```python
from build123d import *

# Parameters (mm, degrees)
SKETCH1_W           = 153
SKETCH1_H           = 100
SKETCH1_R           = 3.25
BOSS_EXTRUDE1_DEPTH = 3.175
CUT_EXTRUDE1_DEPTH  = 92.4457797
CUT_EXTRUDE2_DEPTH  = 92.4457797
FILLET1_R           = 5
SKETCH4_R           = 1.25
CUT_EXTRUDE3_DEPTH  = 92.4457797
SKETCH5_R           = 1.25
CUT_EXTRUDE4_DEPTH  = 92.4457797
SKETCH6_W           = 85
SKETCH6_H           = 12.5
CUT_EXTRUDE5_DEPTH  = 92.4457797


with BuildPart() as part:
    # Sketch1 → Boss-Extrude1 (new body)
    with BuildSketch(Plane(origin=(0, 0, 0), x_dir=(1, 0, 0), z_dir=(0, 1, 0))):
        Rectangle(SKETCH1_W, SKETCH1_H)
        with Locations(Location((-70, 43.5, 0), (0, 0, 270))):
            Circle(SKETCH1_R, mode=Mode.SUBTRACT)
        with Locations(Location((70, 43.5, 0), (0, 0, 270))):
            Circle(SKETCH1_R, mode=Mode.SUBTRACT)
        with Locations(Location((70, -43.5, 0), (0, 0, 270))):
            Circle(SKETCH1_R, mode=Mode.SUBTRACT)
        with Locations(Location((-70, -43.5, 0), (0, 0, 270))):
            Circle(SKETCH1_R, mode=Mode.SUBTRACT)
    extrude(amount=BOSS_EXTRUDE1_DEPTH)

    # Sketch2 → Cut-Extrude1 (cut, through all)
    with BuildSketch(Plane(origin=(0, 3.175, 0), x_dir=(1, 0, 0), z_dir=(0, 1, 0))):
        Polygon((-76.5, 35), (-66.5, 35), (-45, 13.5), (-45, -13.5), (-66.5, -35), (-76.5, -35), align=None)
        Polygon((76.5, -35), (66.5, -35), (45, -13.5), (45, 13.5), (66.5, 35), (76.5, 35), align=None)
    extrude(amount=-CUT_EXTRUDE1_DEPTH, mode=Mode.SUBTRACT)

    # Sketch3 → Cut-Extrude2 (cut, through all)
    with BuildSketch(Plane(origin=(0, 3.175, 0), x_dir=(1, 0, 0), z_dir=(0, 1, 0))):
        with BuildLine():
            Line((-50, 45), (-50, 60))
            ThreePointArc((-50, 60), (-42.5, 67.5), (-35, 60))
            Line((-35, 60), (-35, 45))
            ThreePointArc((-35, 45), (-42.5, 37.5), (-50, 45))
        make_face()
        with BuildLine():
            Line((50, 45), (50, 60))
            ThreePointArc((50, 60), (42.5, 67.5), (35, 60))
            Line((35, 60), (35, 45))
            ThreePointArc((35, 45), (42.5, 37.5), (50, 45))
        make_face()
        with BuildLine():
            Line((-50, -45), (-50, -60))
            ThreePointArc((-50, -60), (-42.5, -67.5), (-35, -60))
            Line((-35, -60), (-35, -45))
            ThreePointArc((-35, -45), (-42.5, -37.5), (-50, -45))
        make_face()
        with BuildLine():
            Line((50, -45), (50, -60))
            ThreePointArc((50, -60), (42.5, -67.5), (35, -60))
            Line((35, -60), (35, -45))
            ThreePointArc((35, -45), (42.5, -37.5), (50, -45))
        make_face()
    extrude(amount=-CUT_EXTRUDE2_DEPTH, mode=Mode.SUBTRACT)

    # Fillet1
    fillet1_edges = [part.edges().sort_by_distance(p)[0] for p in [
        (-45, 1.5875, -13.5),
        (-45, 1.5875, 13.5),
        (-66.5, 1.5875, 35),
        (-50, 1.5875, 50),
        (-35, 1.5875, 50),
        (35, 1.5875, 50),
        (50, 1.5875, 50),
        (66.5, 1.5875, 35),
        (45, 1.5875, 13.5),
        (45, 1.5875, -13.5),
        (66.5, 1.5875, -35),
        (50, 1.5875, -50),
        (35, 1.5875, -50),
        (-35, 1.5875, -50),
        (-50, 1.5875, -50),
        (-66.5, 1.5875, -35),
    ]]
    fillet(fillet1_edges, radius=FILLET1_R - 0.0001)  # a hair under: the kernel refuses the full size

    # Sketch4 → Cut-Extrude3 (cut, through all)
    with BuildSketch(Plane(origin=(0, 3.175, 0), x_dir=(1, 0, 0), z_dir=(0, 1, 0))):
        with Locations(Location((-32.76, 10, 0), (0, 0, 270))):
            Circle(SKETCH4_R)
        with Locations(Location((-14.76, 22, 0), (0, 0, 270))):
            Circle(SKETCH4_R)
        with Locations(Location((-14.76, -22, 0), (0, 0, 270))):
            Circle(SKETCH4_R)
        with Locations(Location((-32.76, -22, 0), (0, 0, 270))):
            Circle(SKETCH4_R)
        with Locations(Location((32.76, -22, 0), (0, 0, 90))):
            Circle(SKETCH4_R)
        with Locations(Location((14.76, -22, 0), (0, 0, 90))):
            Circle(SKETCH4_R)
        with Locations(Location((14.76, 22, 0), (0, 0, 90))):
            Circle(SKETCH4_R)
        with Locations(Location((32.76, 10, 0), (0, 0, 90))):
            Circle(SKETCH4_R)
    extrude(amount=-CUT_EXTRUDE3_DEPTH, mode=Mode.SUBTRACT)

    # Sketch5 → Cut-Extrude4 (cut, through all)
    with BuildSketch(Plane(origin=(0, 3.175, 0), x_dir=(1, 0, 0), z_dir=(0, 1, 0))):
        with Locations(Location((-5, -10, 0), (0, 0, 270))):
            Circle(SKETCH5_R)
        with Locations(Location((5, -10, 0), (0, 0, 270))):
            Circle(SKETCH5_R)
    extrude(amount=-CUT_EXTRUDE4_DEPTH, mode=Mode.SUBTRACT)

    # Sketch6 → Cut-Extrude5 (cut, through all)
    with BuildSketch(Plane(origin=(0, 3.175, 0), x_dir=(1, 0, 0), z_dir=(0, 1, 0))):
        with Locations((0, 43.75)):
            Rectangle(SKETCH6_W, SKETCH6_H)
        with Locations((0, -43.75)):
            Rectangle(SKETCH6_W, SKETCH6_H)
    extrude(amount=-CUT_EXTRUDE5_DEPTH, mode=Mode.SUBTRACT)


solid = part.part
```
Input: part model. Units: mm. Frame: model coordinates. A direction names the side the tool comes from. Give positions to 0.01 mm unless a question says otherwise; leave off trailing zeros. Loops run counter-clockwise (first coordinate to the right, second up) from the corner with the lowest first, then second, coordinate; pieces in that order, holes last. Notation, with made-up numbers: (41.25, -15.5) -> (58.25, -15.5) arc R32 cw to (58.25, 17.5) -> close; hole circle Ø9 at (83, 60). An arc over 180 degrees is marked (long way). Use a Markdown table: item, result.
Q1. Access query for faces 1 (the flat face through (-1, 2, -37.5)), 2 (the cylindrical face through (-52, 2, 49)), 3 (the flat face through (-55.6, 1.6, 24.1)), 4 (the cylindrical face through (66.63, 1.57, 34.61)). Directions: +Z, -Z, +X, -X, +Y, -Y. A direction counts if a zero-diameter tool reaches every point of the face in a straight line with its end or side. Return the directions, or none.
Entries:
| item | result |
|---|---|
| face 1 | -Z, +Y, -Y |
| face 2 | +Z, +Y, -Y |
| face 3 | -X, +Y, -Y |
| face 4 | +X, +Y, -Y |
Q2. Section query B-B, the plane y = 2.25. State how many separate pieces and enclosed holes the cut face has, plus the area to 3 significant figures.
Entries:
| item | result |
|---|---|
| separate pieces | 1 |
| enclosed holes | 14 |
| area | 9,160 mm² |
Q3. Section query C-C, the plane x = 12. Return the cut outline in (y, z) (3 decimals).
Entries:
| item | result |
|---|---|
| outline | (0, -37.5) -> (3.175, -37.5) -> (3.175, 37.5) -> (0, 37.5) -> close |
Q4. First-contact query: P1, Ø1.5, axis at x = -32, y = 2.5, coming from the +Z side. Flat tip, straight axial feed; report the tip coordinate or a pass-through.
Entries:
| item | result |
|---|---|
| P1 | stops at z = 37.5 |
Q5. Pull-direction query (X, two-part tool) for faces 5 (the cylindrical face through (45.39, 1.57, -13.37)), 6 (the flat face through (-72, 2, 35)), 7 (the cylindrical face through (68.755, 1.565, -40.498)); classes: pulls with the +X half, pulls with the -X half, needs draft (parallel to the pull), parting line crosses it, or undercut.
Entries:
| item | result |
|---|---|
| face 5 | pulls with the +X half |
| face 6 | needs draft |
| face 7 | undercut |
Q6. Section query A-A, the plane z = -43.5. Return the cut outline in (x, y) (3 decimals).
Entries:
| item | result |
|---|---|
| outline | (-76.5, 0) -> (-73.25, 0) -> (-73.25, 3.175) -> (-76.5, 3.175) -> close; (-66.75, 0) -> (-49.848, 0) -> (-49.848, 3.175) -> (-66.75, 3.175) -> close; (49.848, 0) -> (66.75, 0) -> (66.75, 3.175) -> (49.848, 3.175) -> close; (73.25, 0) -> (76.5, 0) -> (76.5, 3.175) -> (73.25, 3.175) -> close |
Q7. Ray query, probe 1 along X at (y, z) = (2.55, -10); probe 2 along Z at (x, y) = (32.76, 1.1); probe 3 along X at (y, z) = (1.4, 10). Return the intervals inside material, ascending. Write a range as from..to.
Entries:
| item | result |
|---|---|
| probe 1 | x = -45..-34.01, -31.51..31.51, 34.01..45 |
| probe 2 | z = -37.5..-11.25, -8.75..20.75, 23.25..37.5 |
| probe 3 | x = -45..-6.25, -3.75..3.75, 6.25..45 |
